```python
from build123d import *

# Parameters (mm, degrees)
SKETCH1_R           = 89.6625
SKETCH1_R_2         = 85.865
BOSS_EXTRUDE1_DEPTH = 42.425
SKETCH2_W           = 20
SKETCH2_H           = 11
CUT_EXTRUDE1_DEPTH  = 134.710913681
CIRPATTERN1_COUNT   = 11


with BuildPart() as part:
    # Sketch1 → Boss-Extrude1 (new body)
    with BuildSketch(Plane(origin=(0, 0, 0), x_dir=(1, 0, 0), z_dir=(0, 1, 0))):
        with Locations(Location((0, 0, 0), (0, 0, 90))):
            Circle(SKETCH1_R)
        with Locations(Location((0, 0, 0), (0, 0, 90))):
            Circle(SKETCH1_R_2, mode=Mode.SUBTRACT)
    extrude(amount=BOSS_EXTRUDE1_DEPTH)

    # Sketch2 → Cut-Extrude1 (cut, symmetric)
    with BuildSketch(Plane.XY):
        with Locations((0, 19.5)):
            Rectangle(SKETCH2_W, SKETCH2_H)
    cut_extrude1 = extrude(amount=CUT_EXTRUDE1_DEPTH, both=True, mode=Mode.SUBTRACT)

    # CirPattern1: Cut-Extrude1 ×11 about axis
    cirpattern1_axis = Axis((0, 0, 0), (0, 1, 0))
    for i in range(1, CIRPATTERN1_COUNT):
        add(cut_extrude1.rotate(cirpattern1_axis, i * 360 / CIRPATTERN1_COUNT), mode=Mode.SUBTRACT)


solid = part.part
```
Work out the finished part from the listing and answer in its coordinate system (mm). Give positions to 0.01 mm unless a question says otherwise; leave off trailing zeros. Order: outer loops, then holes, each group sorted by start corner. A loop starts at its lowest first (then second) coordinate and runs counter-clockwise, first axis right, second up.
1. Each of these flat-tipped pins is pushed along its axis until it touches: P1, Ø10, axis at y = 30.5, z = -54.5, coming from the -X side; P2, Ø6, axis at y = 26, z = 54.5, coming from the +X side; P3, Ø3, axis at y = 18, z = 87, coming from the +X side. Where does it stop, or does it pass through?
Result sheet:
P1: stops at x = -74.76
P2: stops at x = 73.4
P3: stops at x = 15.51
2. Section D-D, the plane z = 37 is taken. Determine the outline of the cut face in (x, y) (3 decimals).
Result sheet:
outline: (-81.672, 0) - (-77.484, 0) - (-77.484, 14) - (-81.672, 14) - close; (-81.672, 25) - (-77.484, 25) - (-77.484, 42.425) - (-81.672, 42.425) - close; (77.484, 0) - (81.672, 0) - (81.672, 14) - (77.484, 14) - close; (77.484, 25) - (81.672, 25) - (81.672, 42.425) - (77.484, 42.425) - close
3. Section B-B, the plane z = 0 is taken. Determine the outline of the cut face in (x, y) (1 decimal), and give its area (3 significant figures).
Result sheet:
outline: (-89.7, 0) - (-85.9, 0) - (-85.9, 42.4) - (-89.7, 42.4) - close; (85.9, 0) - (89.7, 0) - (89.7, 42.4) - (85.9, 42.4) - close
area: 322 mm2
4. Straight lines are drawn through the part: L1, parallel to X at y = 16, z = 0 (1 decimal); L2, parallel to X at y = 29, z = -76; L3, parallel to Z at x = -7, y = 3. For each, find the intervals that lie inside material, in ascending order.
Result sheet:
L1: x = -89.7 to -85.9, 85.9 to 89.7
L2: x = -47.57 to -39.96, 39.96 to 47.57
L3: z = -89.39 to -85.58, 85.58 to 89.39
5. Section A-A, the plane x = 0 is taken. Determine the outline of the cut face in (y, z) (1 decimal), and give its area (3 significant figures).
Result sheet:
outline: (0, -89.7) - (14, -89.7) - (14, -85.9) - (0, -85.9) - close; (0, 85.9) - (14, 85.9) - (14, 89.7) - (0, 89.7) - close; (25, -89.7) - (42.4, -89.7) - (42.4, -85.9) - (25, -85.9) - close; (25, 85.9) - (42.4, 85.9) - (42.4, 89.7) - (25, 89.7) - close
area: 239 mm2
6. Section C-C, the plane y = 6.5 is taken. Determine the outline of the cut face in (x, z) (1 decimal).
Result sheet:
outline: circle Ø179.3 at (0, 0); hole circle Ø171.7 at (0, 0)
7. The mould has two halves that part along Z. Classify faces 1 (the cylindrical face through (-72.4, 20.92, -46.16)), 2 (the flat face through (0, 25, -87)): released by +Z, released by -Z, zero draft, split by the parting line, or undercut.
Result sheet:
face 1: undercut
face 2: zero draft
